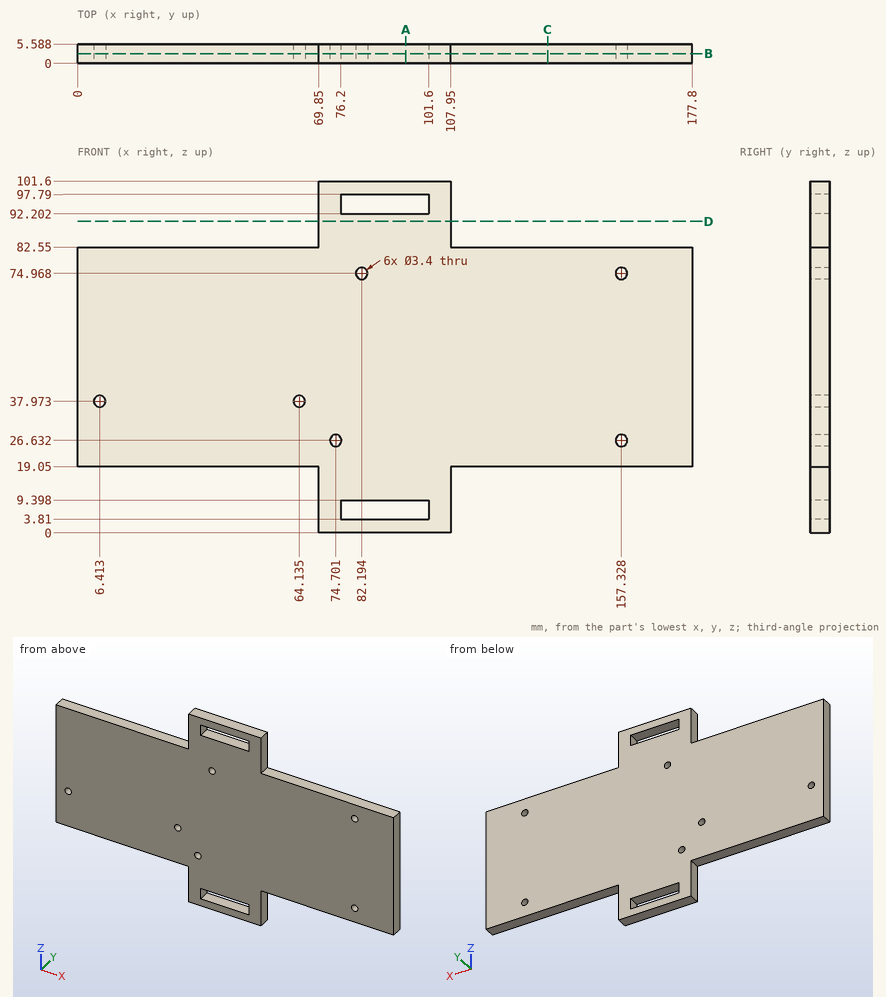
Design review of the part shown in the three views and the two pictorial views. Dimensions are in mm from the part's minimum x, y and z. Give positions to 0.01 mm unless a question says otherwise; leave off trailing zeros. Loops run counter-clockwise (first coordinate to the right, second up) from the corner with the lowest first, then second, coordinate; pieces in that order, holes last. Notation, with made-up numbers: (82, 55.5) - (141, 55.5) arc R21 cw to (141, 59.5) - close; hole circle Ø6 at (35, 17.25). An arc over 180 degrees is marked (long way). Use CSV: the item, a comma, the result in double quotes. Start each with the question number.
1. Add section C-C (x = 136). State the section outline as (y, z) points.
2. Insertion check: P1, Ø1.7, axis at x = 151, y = 3.5, coming from the -Z side; P2, Ø1.7, axis at y = 2.5, z = 94, coming from the +X side; P3, Ø1.7, axis at x = 43.5, y = 2, coming from the +Z side. Each pin has a flat end and moves straight along its axis. Give the tip position at first contact, or say it passes through.
3. Add section B-B (y = 2.8). Count the separate pieces of the cut face and the enclosed holes in it, plus the area to 3 significant figures.
4. Add section A-A (x = 95). State the section outline as (y, z) points.
5. Add section D-D (z = 90). State the section outline as (x, y) points.
6. Wall thickness on L1, parallel to Z at x = 85.5, y = 4.4; L2, parallel to X at y = 5.2, z = 97; L3, parallel to Z at x = 31, y = 4.3: over which ranges is each line inside the solid? List them lowest first.
Results found:
1,outline,"(0, 19.05) - (5.59, 19.05) - (5.59, 82.55) - (0, 82.55) - close"
2,P1,"stops at z = 19.05"
2,P2,"stops at x = 107.95"
2,P3,"stops at z = 82.55"
3,separate pieces,"1"
3,enclosed holes,"8"
3,area,"12,400 mm²"
4,outline,"(0, 0) - (5.59, 0) - (5.59, 3.81) - (0, 3.81) - close; (0, 9.4) - (5.59, 9.4) - (5.59, 92.2) - (0, 92.2) - close; (0, 97.79) - (5.59, 97.79) - (5.59, 101.6) - (0, 101.6) - close"
5,outline,"(69.85, 0) - (107.95, 0) - (107.95, 5.59) - (69.85, 5.59) - close"
6,L1,"z = 0 to 3.81, 9.4 to 92.2, 97.79 to 101.6"
6,L2,"x = 69.85 to 76.2, 101.6 to 107.95"
6,L3,"z = 19.05 to 82.55"
